Can you work these out from the model? Positions are in its coordinate system, mm. Give positions to 0.01 mm unless a question says otherwise; leave off trailing zeros. Loops run counter-clockwise (first coordinate to the right, second up) from the corner with the lowest first, then second, coordinate; pieces in that order, holes last. Notation, with made-up numbers: M 19.25,16.5 L 47.25,16.5 A19 ccw 47.25,26.5 Z; hole C -23.75,25.5 d8. An arc over 180 degrees is marked long. Put each result on its own line as item: value. Start each with the question number.
1) For P1, Ø6, axis at x = 1051.5, z = -134, coming from the +Y side; P2, Ø10, axis at y = 1664.5, z = -156.5, coming from the -X side (3 decimals); P3, Ø2, axis at x = 1010, z = -184, coming from the -Y side; P4, Ø6, axis at x = 1054, z = -201.5, coming from the +Y side, each with a flat end and sliding along its axis, tell me the tip position at first contact or that it passes through.
2) Please list where these lines run through material, in increasing order: line 1 along Z through (x, y) = (1016.5, 1348); line 2 along Z through (x, y) = (1046, 1846); line 3 along Y through (x, z) = (1018.5, -232). Write a range as from..to.
3) Imagine slicing it at C-C (z = -149.5). Write out the boundary of the cut face in (x, y), then the cut area to 3 significant figures.
4) Imagine slicing it at A-A (y = 1694.5). Write out the boundary of the cut face in (x, z), then the cut area to 3 significant figures.
5) Imagine slicing it at D-D (z = -113). Write out the boundary of the cut face in (x, y), then the cut area to 3 significant figures.
6) Imagine slicing it at B-B (x = 1056). Write out the boundary of the cut face in (y, z), then the cut area to 3 significant figures.
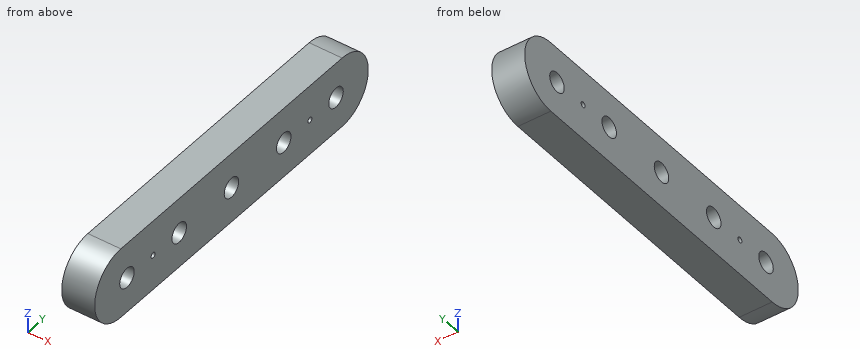
from build123d import *

# Parameters (mm, degrees)
BOSS_EXTRUDE1_DEPTH = 76.2
CUT_EXTRUDE1_REACH  = 78.2
SKETCH3_R           = 22.86
CUT_EXTRUDE2_REACH  = 78.2
SKETCH4_R           = 6.35


with BuildPart() as part:
    # Sketch2 → Boss-Extrude1 (new body)
    with BuildSketch(Plane.ZY.offset(-1066.346797213)):
        with BuildLine():
            Line((-82.55, 1331.163756946), (-82.55, 2028.051006195))
            ThreePointArc((-82.55, 2028.051006195), (-164.799803954, 2110.300810149), (-247.049607907, 2028.051006195))
            Line((-247.049607907, 2028.051006195), (-247.049607907, 1331.163756946))
            ThreePointArc((-247.049607907, 1331.163756946), (-164.799803954, 1248.913952992), (-82.55, 1331.163756946))
        make_face()
    extrude(amount=BOSS_EXTRUDE1_DEPTH)

    # Sketch3 → Cut-Extrude1 (cut, up to next)
    with BuildSketch(Plane(origin=(1066.346797213, 0, 0), x_dir=(0, 0, -1), z_dir=(1, 0, 0)), mode=Mode.PRIVATE) as cut_extrude1_sk1:
        with Locations((164.799803954, 1844.15409586)):
            Circle(SKETCH3_R)
    cut_extrude1_tool1 = extrude(cut_extrude1_sk1.sketch, amount=-CUT_EXTRUDE1_REACH, mode=Mode.PRIVATE) & part.part
    add(cut_extrude1_tool1.solids().sort_by_distance((1066.346797, 1844.154096, -164.799804))[0], mode=Mode.SUBTRACT)
    # Sketch3 → Cut-Extrude1 (cut, up to next)
    with BuildSketch(Plane(origin=(1066.346797213, 0, 0), x_dir=(0, 0, -1), z_dir=(1, 0, 0)), mode=Mode.PRIVATE) as cut_extrude1_sk2:
        with Locations((164.799803954, 1679.607381571)):
            Circle(SKETCH3_R)
    cut_extrude1_tool2 = extrude(cut_extrude1_sk2.sketch, amount=-CUT_EXTRUDE1_REACH, mode=Mode.PRIVATE) & part.part
    add(cut_extrude1_tool2.solids().sort_by_distance((1066.346797, 1679.607382, -164.799804))[0], mode=Mode.SUBTRACT)
    # Sketch3 → Cut-Extrude1 (cut, up to next)
    with BuildSketch(Plane(origin=(1066.346797213, 0, 0), x_dir=(0, 0, -1), z_dir=(1, 0, 0)), mode=Mode.PRIVATE) as cut_extrude1_sk3:
        with Locations((164.799803954, 2008.700810149)):
            Circle(SKETCH3_R)
    cut_extrude1_tool3 = extrude(cut_extrude1_sk3.sketch, amount=-CUT_EXTRUDE1_REACH, mode=Mode.PRIVATE) & part.part
    add(cut_extrude1_tool3.solids().sort_by_distance((1066.346797, 2008.70081, -164.799804))[0], mode=Mode.SUBTRACT)
    # Sketch3 → Cut-Extrude1 (cut, up to next)
    with BuildSketch(Plane(origin=(1066.346797213, 0, 0), x_dir=(0, 0, -1), z_dir=(1, 0, 0)), mode=Mode.PRIVATE) as cut_extrude1_sk4:
        with Locations((164.799803954, 1515.060667281)):
            Circle(SKETCH3_R)
    cut_extrude1_tool4 = extrude(cut_extrude1_sk4.sketch, amount=-CUT_EXTRUDE1_REACH, mode=Mode.PRIVATE) & part.part
    add(cut_extrude1_tool4.solids().sort_by_distance((1066.346797, 1515.060667, -164.799804))[0], mode=Mode.SUBTRACT)
    # Sketch3 → Cut-Extrude1 (cut, up to next)
    with BuildSketch(Plane(origin=(1066.346797213, 0, 0), x_dir=(0, 0, -1), z_dir=(1, 0, 0)), mode=Mode.PRIVATE) as cut_extrude1_sk5:
        with Locations((164.799803954, 1350.513952992)):
            Circle(SKETCH3_R)
    cut_extrude1_tool5 = extrude(cut_extrude1_sk5.sketch, amount=-CUT_EXTRUDE1_REACH, mode=Mode.PRIVATE) & part.part
    add(cut_extrude1_tool5.solids().sort_by_distance((1066.346797, 1350.513953, -164.799804))[0], mode=Mode.SUBTRACT)

    # Sketch4 → Cut-Extrude2 (cut, up to next)
    with BuildSketch(Plane(origin=(1066.346797213, 0, 0), x_dir=(0, 0, -1), z_dir=(1, 0, 0)), mode=Mode.PRIVATE) as cut_extrude2_sk1:
        with Locations((164.799803954, 1926.427453004)):
            Circle(SKETCH4_R)
    cut_extrude2_tool1 = extrude(cut_extrude2_sk1.sketch, amount=-CUT_EXTRUDE2_REACH, mode=Mode.PRIVATE) & part.part
    add(cut_extrude2_tool1.solids().sort_by_distance((1066.346797, 1926.427453, -164.799804))[0], mode=Mode.SUBTRACT)
    # Sketch4 → Cut-Extrude2 (cut, up to next)
    with BuildSketch(Plane(origin=(1066.346797213, 0, 0), x_dir=(0, 0, -1), z_dir=(1, 0, 0)), mode=Mode.PRIVATE) as cut_extrude2_sk2:
        with Locations((164.799803954, 1432.787310137)):
            Circle(SKETCH4_R)
    cut_extrude2_tool2 = extrude(cut_extrude2_sk2.sketch, amount=-CUT_EXTRUDE2_REACH, mode=Mode.PRIVATE) & part.part
    add(cut_extrude2_tool2.solids().sort_by_distance((1066.346797, 1432.78731, -164.799804))[0], mode=Mode.SUBTRACT)


solid = part.part
Recorded:
1. P1: y = 2105.46
1. P2: through
1. P3: y = 1250.95
1. P4: y = 2103.08
2. line 1: -247.05..-187.52, -142.08..-82.55
2. line 2: -247.05..-187.59, -142.01..-82.55
2. line 3: 1283.74..2075.48
3. outline: M 990.15,1250.35 L 1066.35,1250.35 L 1066.35,1333.53 L 990.15,1333.53 Z; M 990.15,1367.5 L 1066.35,1367.5 L 1066.35,1498.08 L 990.15,1498.08 Z; M 990.15,1532.05 L 1066.35,1532.05 L 1066.35,1662.62 L 990.15,1662.62 Z; M 990.15,1696.59 L 1066.35,1696.59 L 1066.35,1827.17 L 990.15,1827.17 Z; M 990.15,1861.14 L 1066.35,1861.14 L 1066.35,1991.72 L 990.15,1991.72 Z; M 990.15,2025.69 L 1066.35,2025.69 L 1066.35,2108.87 L 990.15,2108.87 Z
3. area: 52,500 mm²
4. outline: M 990.15,-247.05 L 1066.35,-247.05 L 1066.35,-182.14 L 990.15,-182.14 Z; M 990.15,-147.46 L 1066.35,-147.46 L 1066.35,-82.55 L 990.15,-82.55 Z
4. area: 9,890 mm²
5. outline: M 990.15,1267.27 L 1066.35,1267.27 L 1066.35,2091.94 L 990.15,2091.94 Z
5. area: 62,800 mm²
6. outline: M 1331.16,-247.05 L 2028.05,-247.05 A82.25 ccw 2028.05,-82.55 L 1331.16,-82.55 A82.25 ccw Z; hole C 1350.51,-164.8 d45.72; hole C 1432.79,-164.8 d12.7; hole C 1515.06,-164.8 d45.72; hole C 1679.61,-164.8 d45.72; hole C 1844.15,-164.8 d45.72; hole C 1926.43,-164.8 d12.7; hole C 2008.7,-164.8 d45.72
6. area: 127,000 mm²
